Source: CAD feature listing. Evaluate the final solid. Frame: model axes, mm. A direction names the side the tool comes from. Give positions to 0.01 mm unless a question says otherwise; leave off trailing zeros. Loops run counter-clockwise (first coordinate to the right, second up) from the corner with the lowest first, then second, coordinate; pieces in that order, holes last.
```python
from build123d import *

# Parameters (mm, degrees)
SKETCH_1_W           = 52
SKETCH_1_H           = 28
EXTRUDE_1_DEPTH      = 1.55
FILLET_1_R           = 1
SKETCH_2_W           = 37.76
SKETCH_2_H           = 2.54
EXTRUDE_2_DEPTH      = 2.54
SKETCH_3_W           = 17.5
SKETCH_3_H           = 15.75
EXTRUDE_4_DEPTH      = 2.4
EXTRUDE_6_DEPTH      = 1.8
EXTRUDE_6_DEPTH_BACK = 5.6
SKETCH1_R            = 0.9
SKETCH1_W            = 3
SKETCH1_H            = 4
BOSS_EXTRUDE1_DEPTH  = 1.4
SKETCH1_4_R          = 0.9
BOSS_EXTRUDE2_DEPTH  = 1.95
SKETCH2_W            = 0.9
SKETCH2_H            = 1.75
BOSS_EXTRUDE3_DEPTH  = 0.64


with BuildPart() as part:
    # Sketch 1 → Extrude 1 (new body)
    with BuildSketch(Plane(origin=(0, 0, 0), x_dir=(1, 0, 0), z_dir=(0, 1, 0))):
        Rectangle(SKETCH_1_W, SKETCH_1_H)
    extrude(amount=EXTRUDE_1_DEPTH)

    # Fillet 1
    fillet_1_edges = [part.edges().sort_by_distance(p)[0] for p in [
        (26, 0.775, 14),
        (-26, 0.775, 14),
        (-26, 0.775, -14),
        (26, 0.775, -14),
    ]]
    fillet(fillet_1_edges, radius=FILLET_1_R)

    # Sketch 2 → Extrude 2 (add)
    with BuildSketch(Plane.XZ):
        with Locations((1.27, 12.73)):
            Rectangle(SKETCH_2_W, SKETCH_2_H)
        with Locations((1.27, -12.73)):
            Rectangle(SKETCH_2_W, SKETCH_2_H)
    extrude(amount=EXTRUDE_2_DEPTH)

    # Sketch 3 → Extrude 4 (add)
    with BuildSketch(Plane(origin=(0, 1.55, 0), x_dir=(1, 0, 0), z_dir=(0, 1, 0))):
        with Locations((10.35, 0)):
            Rectangle(SKETCH_3_W, SKETCH_3_H)
    extrude(amount=EXTRUDE_4_DEPTH)

    # Sketch 5 → Extrude 6 (add, two sides)
    with BuildSketch(Plane.ZY.offset(26)) as extrude_6_sk:
        with BuildLine():
            Line((7.35, 1.55), (0.87, 1.55))
            ThreePointArc((0.87, 1.55), (-0.013883476, 1.916116524), (-0.38, 2.8))
            Line((-0.38, 2.8), (-0.38, 3.58))
            ThreePointArc((-0.38, 3.58), (-0.013883476, 4.463883476), (0.87, 4.83))
            Line((0.87, 4.83), (7.35, 4.83))
            ThreePointArc((7.35, 4.83), (8.233883476, 4.463883476), (8.6, 3.58))
            Line((8.6, 3.58), (8.6, 2.8))
            ThreePointArc((8.6, 2.8), (8.233883476, 1.916116524), (7.35, 1.55))
        make_face()
    extrude(amount=EXTRUDE_6_DEPTH)
    extrude(extrude_6_sk.sketch, amount=-EXTRUDE_6_DEPTH_BACK)

    # Sketch1 → Boss-Extrude1 (add)
    with BuildSketch(Plane(origin=(0, 1.55, 0), x_dir=(1, 0, 0), z_dir=(0, 1, 0))):
        with Locations((-16.3, -3.33)):
            Circle(SKETCH1_R)
        with Locations((-16.3, -3.33)):
            Rectangle(SKETCH1_W, SKETCH1_H)
        with Locations((-16.3, -3.33)):
            Circle(SKETCH1_R, mode=Mode.SUBTRACT)
    extrude(amount=BOSS_EXTRUDE1_DEPTH)

    # Sketch1_4 → Boss-Extrude2 (add)
    with BuildSketch(Plane(origin=(0, 1.55, 0), x_dir=(1, 0, 0), z_dir=(0, 1, 0))):
        with Locations((-16.3, -3.33)):
            Circle(SKETCH1_4_R)
    extrude(amount=BOSS_EXTRUDE2_DEPTH)

    # Sketch2 → Boss-Extrude3 (add)
    with BuildSketch(Plane(origin=(0, 1.55, 0), x_dir=(1, 0, 0), z_dir=(0, 1, 0))):
        with Locations((-19.24, 11.015)):
            Rectangle(SKETCH2_W, SKETCH2_H)
        with Locations((-3.11, 0.305)):
            Rectangle(SKETCH2_W, SKETCH2_H)
        with Locations((-3.11, -4.885)):
            Rectangle(SKETCH2_W, SKETCH2_H)
    extrude(amount=BOSS_EXTRUDE3_DEPTH)


solid = part.part
```
(1) Section C-C, the plane z = -6. Return the cut outline in (x, y), then the cut area to 3 significant figures.
A:
outline: (-26, 0) - (26, 0) - (26, 1.55) - (19.1, 1.55) - (19.1, 3.95) - (1.6, 3.95) - (1.6, 1.55) - (-26, 1.55) - close
area: 123 mm2
(2) Section D-D, the plane z = 3.33. Return the cut outline in (x, y), then the cut area to 3 significant figures.
A:
outline: (-27.8, 1.55) - (-26, 1.55) - (-26, 0) - (26, 0) - (26, 1.55) - (19.1, 1.55) - (19.1, 3.95) - (1.6, 3.95) - (1.6, 1.55) - (-14.8, 1.55) - (-14.8, 2.95) - (-15.4, 2.95) - (-15.4, 3.5) - (-17.2, 3.5) - (-17.2, 2.95) - (-17.8, 2.95) - (-17.8, 1.55) - (-20.4, 1.55) - (-20.4, 4.83) - (-27.8, 4.83) - close
area: 152 mm2
(3) Section A-A, the plane y = -1.5. Return the cut outline in (x, z), then the cut area to 3 significant figures.
A:
outline: (-17.61, -14) - (20.15, -14) - (20.15, -11.46) - (-17.61, -11.46) - close; (-17.61, 11.46) - (20.15, 11.46) - (20.15, 14) - (-17.61, 14) - close
area: 192 mm2
(4) Section B-B, the plane x = -16.3. Return the cut outline in (y, z).
A:
outline: (-2.54, -14) - (1.55, -14) - (1.55, 1.33) - (2.95, 1.33) - (2.95, 2.43) - (3.5, 2.43) - (3.5, 4.23) - (2.95, 4.23) - (2.95, 5.33) - (1.55, 5.33) - (1.55, 14) - (-2.54, 14) - (-2.54, 11.46) - (0, 11.46) - (0, -11.46) - (-2.54, -11.46) - close
(5) First-contact query: pin 1 (8 mm diameter, centred on x = -0.5, z = -5.5, fed in from +Y); pin 2 (8.5 mm diameter, centred on x = -1, z = 3, fed in from -Y); pin 3 (1.5 mm diameter, centred on x = 12.5, z = -9.5, fed in from +Y). Flat tips, straight axial feed; report the tip coordinate or a pass-through.
A:
pin 1: stops at y = 3.95
pin 2: stops at y = 0
pin 3: stops at y = 1.55
(6) Ray query, line 1 along X through (y, z) = (1.75, 3.25); line 2 along Z through (x, y) = (-2, -1.75); line 3 along X through (y, z) = (3.5, 6.5). Return the intervals inside material, ascending.
A:
line 1: x = -27.8 to -20.4, -17.8 to -14.8, 1.6 to 19.1
line 2: z = -14 to -11.46, 11.46 to 14
line 3: x = -27.8 to -20.4, 1.6 to 19.1
(7) Mould query, pull axis X, two halves, no side actions, for faces 1 (the flat face through (1, -2.54, 13)), 2 (the cylindrical face through (-25.715, 0.786, -13.699)), 3 (the flat face through (-16, 2, 5.33)). Classes: pulls with the +X half, pulls with the -X half, needs draft (parallel to the pull), parting line crosses it, or undercut.
A:
face 1: needs draft
face 2: pulls with the -X half
face 3: undercut
(8) Reachability of faces 4 (the flat face through (-17.61, -1, 13)), 5 (the flat face through (1.6, 3, 0)), 6 (the flat face through (10, 3.95, 0)) from +Z, -Z, +X, -X, +Y, -Y: full face, straight path, thin tool, end or side. Return the list, or none.
A:
face 4: +Z, -Z, -X, -Y
face 5: +Z, -Z, +Y
face 6: +Z, -Z, +X, +Y
